The model under review builds one solid part; all positions refer to its coordinate system, in mm. Give positions to 0.01 mm unless a question says otherwise; leave off trailing zeros. Order: outer loops, then holes, each group sorted by start corner. A loop starts at its lowest first (then second) coordinate and runs counter-clockwise, first axis right, second up. Notation, with made-up numbers: (8, 65.25) - (41, 65.25) arc R27 ccw to (41, 101.25) - close; hole circle Ø7 at (15.25, 14). An arc over 180 degrees is marked (long way). Answer as CSV lines item,"result". Start each with the question number.
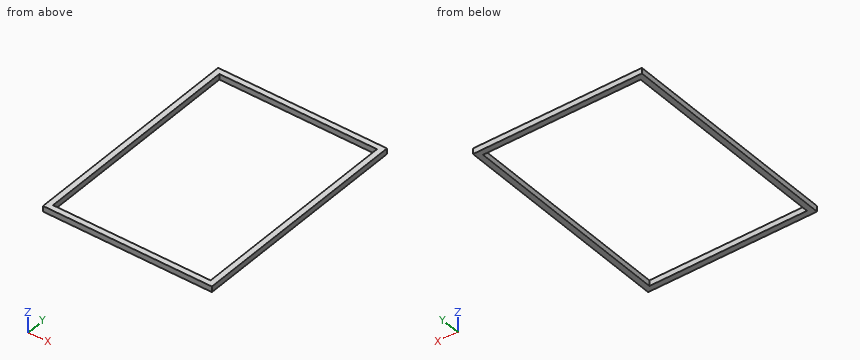
Autodesk Inventor part; units mm, degrees
ref_plane "YZ Plane" through (0, 0, 0) normal (1, 0, 0) x (0, 1, 0)
ref_plane "XZ Plane" through (0, 0, 0) normal (0, 1, 0) x (-1, 0, 0)
ref_plane "XY Plane" through (0, 0, 0) normal (0, 0, 1) x (1, 0, 0)
sketch "Sketch1" plane through (0, 0, 0) normal (0, 0, 1) x (1, 0, 0)
  line L0 (-127.5, 275) -> (172.5, 275)
  line L1 (172.5, 275) -> (172.5, -125)
  line L2 (172.5, -125) -> (-127.5, -125)
  line L3 (-127.5, -125) -> (-127.5, 275)
  line L4 (-117.5, 265) -> (162.5, 265)
  line L5 (162.5, 265) -> (162.5, -115)
  line L6 (162.5, -115) -> (-117.5, -115)
  line L7 (-117.5, -115) -> (-117.5, 265)
  point P0 (0, 0)
  dimension "d0" = 300
  dimension "d1" = 10
  dimension "d2" = 10
  dimension "d3" = 10
  dimension "d4" = 10
  dimension "d5" = 400
  dimension "d6" = 172.5
  dimension "d7" = 115
extrude "Extrusion1" add sketch "Sketch1" along normal mid plane 10
properties part number "Steel support4" material "Steel"
Item 1: Take a section at A-A on y = 186.5. Write out the cut boundary in (x, z).
Item 2: Take a section at B-B on z = 2.75. Write out the cut boundary in (x, y).
Item 3: Take a section at C-C on x = -64.5. Write out the cut boundary in (y, z), and give its area (3 significant figures).
Item 4: For line 1 along Y through (x, z) = (10, -0.25); line 2 along X through (y, z) = (96.5, 0.5), list the stretches that pass through material, from the lowest coordinate up.
Data:
1,outline,"(-127.5, -5) - (-117.5, -5) - (-117.5, 5) - (-127.5, 5) - close; (162.5, -5) - (172.5, -5) - (172.5, 5) - (162.5, 5) - close"
2,outline,"(-127.5, -125) - (172.5, -125) - (172.5, 275) - (-127.5, 275) - close; hole (-117.5, -115) - (162.5, -115) - (162.5, 265) - (-117.5, 265) - close"
3,outline,"(-125, -5) - (-115, -5) - (-115, 5) - (-125, 5) - close; (265, -5) - (275, -5) - (275, 5) - (265, 5) - close"
3,area,"200 mm^2"
4,line 1,"y = -125 to -115, 265 to 275"
4,line 2,"x = -127.5 to -117.5, 162.5 to 172.5"
